Model file for the job. Use its own axes, mm. Coordinates: 2 decimals unless noted, no trailing zeros. Write each loop counter-clockwise with the first axis right and the second up, starting at its lowest first coordinate (ties: lowest second). Pieces come first, ordered by that corner, then holes. Notation, with made-up numbers: (8, -36) -> (54, -36) arc R11 ccw to (54, -17) -> close; hole circle Ø5 at (51.25, 7.25). An arc over 180 degrees is marked (long way). Write item = value, one per line. Start each with the question number.
from build123d import *

# Parameters (mm, degrees)
BOSS_EXTRUDE1_DEPTH = 939.8
SKETCH2_R           = 3.556
CUT_EXTRUDE1_DEPTH  = 941.207951624
FILLET1_R           = 1
FILLET2_R           = 2
SKETCH4_R           = 3.5687
CUT_EXTRUDE2_DEPTH  = 941.23360821


with BuildPart() as part:
    # Sketch1 → Boss-Extrude1 (new body)
    with BuildSketch(Plane(origin=(0, 0, 0), x_dir=(0, 0, -1), z_dir=(1, 0, 0))):
        Polygon((7.856463982, 11.336121381), (7.856463982, -4.538878619), (23.731463982, -4.538878619), (23.731463982, -2.938678619), (9.456663982, -2.938678619), (9.456663982, 11.336121381), align=None)
    extrude(amount=BOSS_EXTRUDE1_DEPTH)

    # Sketch2 → Cut-Extrude1 (cut, through all)
    with BuildSketch(Plane(origin=(0, -2.938678619, 0), x_dir=(1, 0, 0), z_dir=(0, 1, 0))):
        with Locations(Location((12.7, 15.793963982, 0), (0, 0, 270))):
            Circle(SKETCH2_R)
        with Locations(Location((38.1, 15.793963982, 0), (0, 0, 270))):
            Circle(SKETCH2_R)
        with Locations(Location((927.1, 15.793963982, 0), (0, 0, 270))):
            Circle(SKETCH2_R)
        with Locations(Location((901.7, 15.793963982, 0), (0, 0, 270))):
            Circle(SKETCH2_R)
    extrude(amount=-CUT_EXTRUDE1_DEPTH, mode=Mode.SUBTRACT)

    # Fillet1
    fillet1_edges = [part.edges().sort_by_distance(p)[0] for p in [
        (469.9, 11.336121381, -9.456663982),
        (469.9, -2.938678619, -23.731463982),
    ]]
    fillet(fillet1_edges, radius=FILLET1_R)

    # Fillet2
    fillet2_edges = [part.edges().sort_by_distance(p)[0] for p in [
        (469.9, -2.938678619, -9.456663982),
    ]]
    fillet(fillet2_edges, radius=FILLET2_R)

    # Sketch4 → Cut-Extrude2 (cut, through all)
    with BuildSketch(Plane.XZ.offset(4.538878619)):
        with Locations((469.900000001, -20.233163939)):
            Circle(SKETCH4_R)
    extrude(amount=-CUT_EXTRUDE2_DEPTH, mode=Mode.SUBTRACT)


solid = part.part
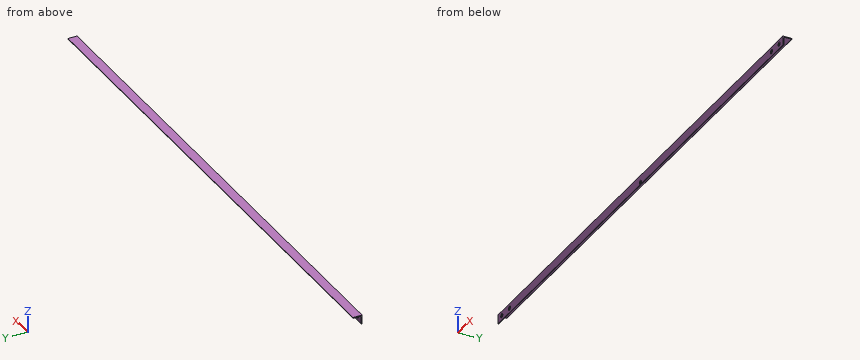
(1) Saw through at A-A (x = 305.5). Give the cut face in (y, z), then the cut area to 3 significant figures.
(2) Drill centre lines: line 1 along Z through (x, y) = (927.1, -4.1); line 2 along Y through (x, z) = (490, -17); line 3 along Z through (x, y) = (712, 2.25). Where is each one in solid material? Low to high.
(3) Saw through at B-B (y = 4.75). Give the cut face in (x, z), then the cut area to 3 significant figures.
(4) Drop flat-ended pins along their axis: pin 1 Ø6 at (x, y) = (812, 2) entering from -Z; pin 2 Ø9 at (x, z) = (470.5, -15.5) entering from +Y. Give the stop position or say it passes through.
Returned:
q1.outline = (-4.54, -23.73) -> (-3.94, -23.73) arc R1 ccw to (-2.94, -22.73) -> (-2.94, -11.46) arc R2 cw to (-0.94, -9.46) -> (10.34, -9.46) arc R1 ccw to (11.34, -8.46) -> (11.34, -7.86) -> (-4.54, -7.86) -> close
q1.area = 48.7 mm2
q2.line_1 = -23.73 to -19.35, -12.24 to -7.86
q2.line_2 = -4.54 to -2.94
q2.line_3 = -9.46 to -7.86
q3.outline = (0, -9.46) -> (939.8, -9.46) -> (939.8, -7.86) -> (0, -7.86) -> close
q3.area = 1,500 mm2
q4.pin_1 = -9.46
q4.pin_2 = -2.89
